from build123d import *

# Parameters (mm, degrees)
F1_DEPTH = 12
F3_D     = 6.5
F5_D     = 6


with BuildPart() as f1:
    # F0 (on Top) → F1 (new body)
    with BuildSketch(Plane.XY):
        Polygon((-25.710834, 25), (-25.710834, 0), (-25.710834, -25), (11.289166, -25), (11.289166, -15), (-5.710834, -15), (-5.710834, 0), (-5.710834, 15), (11.289166, 15), (11.289166, 25), align=None)
    extrude(amount=F1_DEPTH)

    # F3 (through all)
    with Locations(Plane.XY.offset(12)):
        with Locations((-17.710834, -15), (-17.710834, 0), (-17.710834, 15)):
            Hole(F3_D / 2)

    # F5 (through all)
    with Locations(Plane.XZ.offset(25)):
        with Locations((5.289166, 6)):
            Hole(F5_D / 2)


solid = f1.part
Geometry check sheet. Reference: the model listing, model coordinates, mm. A direction names the side the tool comes from. Give positions to 0.01 mm unless a question says otherwise; leave off trailing zeros. Write each loop counter-clockwise with the first axis right and the second up, starting at its lowest first coordinate (ties: lowest second). Pieces come first, ordered by that corner, then holes. Notation, with made-up numbers: (-2, 28.25) - (20, 28.25) arc R26 cw to (20, 43.25) - close; hole circle Ø2 at (22.5, 78). An arc over 180 degrees is marked (long way). Put each result on its own line as item: value.
1. Go/stop test with a flat-tipped pin: pin 1 (2 mm diameter, centred on y = 0, z = 4.5, fed in from +X). Record where the tip stops, or that it passes through.
Ans:
pin 1: stops at x = -5.71
2. Thickness scan on line 1 (Y direction, x = -17.5, z = 4.5); line 2 (Y direction, x = -1.5, z = 7.5); line 3 (Y direction, x = -20.5, z = 9.75). Record the ranges inside material, lowest first.
Ans:
line 1: y = -25 to -18.24, -11.76 to -3.24, 3.24 to 11.76, 18.24 to 25
line 2: y = -25 to -15, 15 to 25
line 3: y = -25 to -16.67, -13.33 to -1.67, 1.67 to 13.33, 16.67 to 25
3. Sectioned sample at C-C, the plane x = -16. Enter the section's corners in (y, z), plus the area to 3 significant figures.
Ans:
outline: (-25, 0) - (-17.76, 0) - (-17.76, 12) - (-25, 12) - close; (-12.24, 0) - (-2.76, 0) - (-2.76, 12) - (-12.24, 12) - close; (2.76, 0) - (12.24, 0) - (12.24, 12) - (2.76, 12) - close; (17.76, 0) - (25, 0) - (25, 12) - (17.76, 12) - close
area: 401 mm²
4. Sectioned sample at A-A, the plane z = 6. Enter the section's corners in (x, y), plus the area to 3 significant figures.
Ans:
outline: (-25.71, -25) - (2.29, -25) - (2.29, -15) - (-5.71, -15) - (-5.71, 15) - (2.29, 15) - (2.29, 25) - (-25.71, 25) - close; (8.29, -25) - (11.29, -25) - (11.29, -15) - (8.29, -15) - close; (8.29, 15) - (11.29, 15) - (11.29, 25) - (8.29, 25) - close; hole circle Ø6.5 at (-17.71, -15); hole circle Ø6.5 at (-17.71, 0); hole circle Ø6.5 at (-17.71, 15)
area: 1,120 mm²
5. Sectioned sample at D-D, the plane z = 11.25. Enter the section's corners in (x, y).
Ans:
outline: (-25.71, -25) - (11.29, -25) - (11.29, -15) - (-5.71, -15) - (-5.71, 15) - (11.29, 15) - (11.29, 25) - (-25.71, 25) - close; hole circle Ø6.5 at (-17.71, -15); hole circle Ø6.5 at (-17.71, 0); hole circle Ø6.5 at (-17.71, 15)
6. Set-up check for faces 1 (the flat face through (1, -15, 6)), 2 (the flat face through (11.289, -20, 6)): record each of +Z, -Z, +X, -X, +Y, -Y from which the full face is reachable in a straight line by a thin tool's end or side.
Ans:
face 1: +Z, -Z, +X
face 2: +Z, -Z, +X, +Y, -Y
7. Sectioned sample at B-B, the plane x = -5. Enter the section's corners in (y, z).
Ans:
outline: (-25, 0) - (-15, 0) - (-15, 12) - (-25, 12) - close; (15, 0) - (25, 0) - (25, 12) - (15, 12) - close
8. Draft check along Y on faces 3 (the flat face through (-7, 25, 6)), 4 (the flat face through (1, 15, 6)), 5 (the flat face through (11.289, 20, 6)), 6 (the flat face through (-5.711, 0, 6)). Enter one of: +Y half, -Y half, draft (parallel to the pull), parting line (faces both ways), or undercut.
Ans:
face 3: +Y half
face 4: undercut
face 5: draft
face 6: undercut
